Here's the drawing with two shaded views (mm, measured from the low corner). I have some questions. Coordinates: 2 decimals unless noted, no trailing zeros. Write each loop counter-clockwise with the first axis right and the second up, starting at its lowest first coordinate (ties: lowest second). Pieces come first, ordered by that corner, then holes. Notation, with made-up numbers: (-6.5, 11.5) -> (0.5, 11.5) arc R23 cw to (0.5, 49.5) -> close; hole circle Ø6 at (32.5, 13). An arc over 180 degrees is marked (long way). Use one line per item in the form item = value.
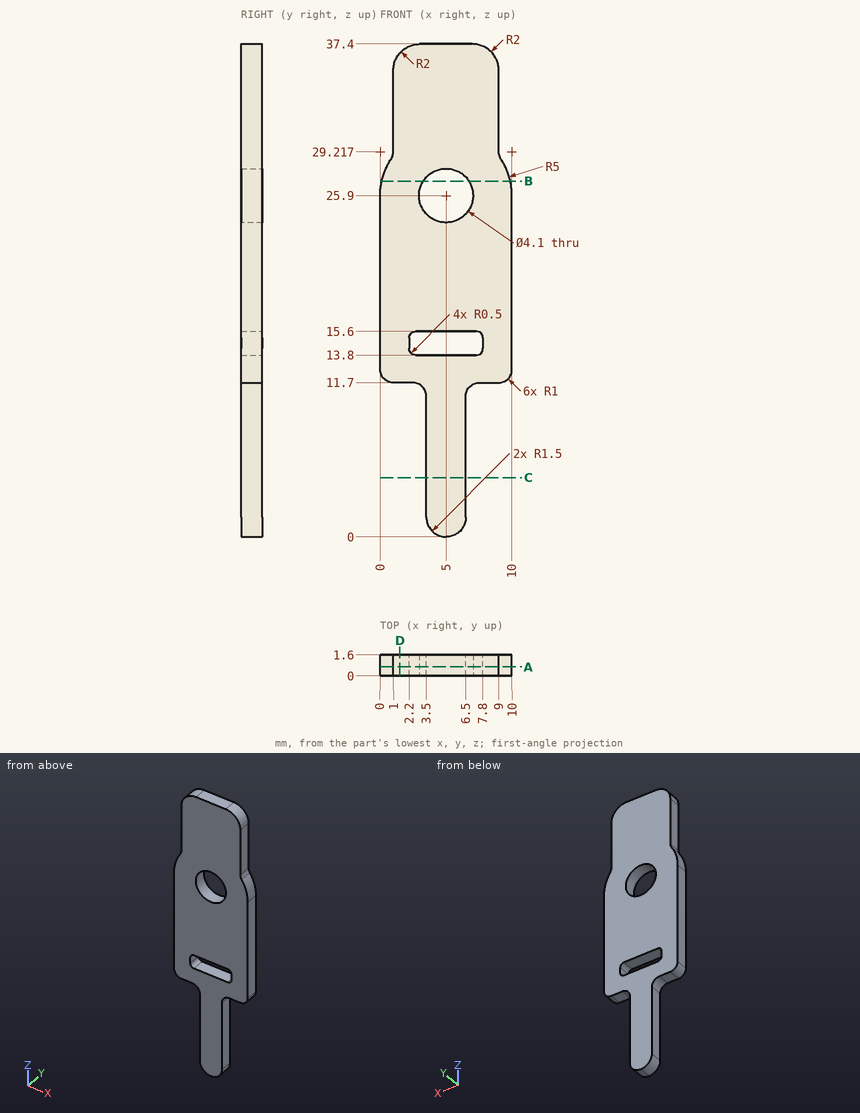
Q1. Suppose I cut it at B-B (z = 27). Write out the boundary of the cut face in (x, y), then the cut area to 3 significant figures.
Return value:
outline = (0.12, 0) -> (3.27, 0) -> (3.27, 1.6) -> (0.12, 1.6) -> close; (6.73, 0) -> (9.88, 0) -> (9.88, 1.6) -> (6.73, 1.6) -> close
area = 10.1 mm2
Q2. Suppose I cut it at C-C (z = 4.5). Write out the boundary of the cut face in (x, y).
Return value:
outline = (3.5, 0) -> (6.5, 0) -> (6.5, 1.6) -> (3.5, 1.6) -> close
Q3. Suppose I cut it at D-D (x = 1.5). Write out the boundary of the cut face in (y, z).
Return value:
outline = (0, 11.7) -> (1.6, 11.7) -> (1.6, 36.72) -> (0, 36.72) -> close
Q4. Suppose I cut it at A-A (y = 0.7). Give the number of separate pieces and of enclosed holes in the cut face.
Return value:
separate_pieces = 1
enclosed_holes = 2
Q5. Will these pins go through, and if not, where does the flat tip stop? pin 1 (0.5 mm diameter, centred on y = 1, z = 4.5, fed in from +X); pin 2 (0.5 mm diameter, centred on y = 1, z = 4, fed in from -X); pin 3 (0.5 mm diameter, centred on y = 1, z = 32.5, fed in from -X).
Return value:
pin_1 = 6.5
pin_2 = 3.5
pin_3 = 1
Q6. If I drill on line 1 (X direction, y = 0.7, z = 25.9); line 2 (Z direction, x = 4.5, y = 0.7) (1 decimal); line 3 (Z direction, x = 4.75, y = 1.5) (1 decimal), over which ranges is the centre line in solid material (lowest first)? Write a range as from..to.
Return value:
line_1 = 0..2.95, 7.05..10
line_2 = 0.1..13.8, 15.6..23.9, 27.9..37.4
line_3 = 0..13.8, 15.6..23.9, 27.9..37.4
